Source: three-view drawing plus pictorial views. Frame: mm from the lowest corner of the part. Round coordinates to 2 decimals unless told otherwise and drop trailing zeros. Write each loop counter-clockwise with the first axis right and the second up, starting at its lowest first coordinate (ties: lowest second). Pieces come first, ordered by that corner, then holes. Notation, with made-up numbers: (54.25, 88.5) -> (112.25, 88.5) arc R12 cw to (112.25, 101.5) -> close; hole circle Ø7 at (1.25, 38). An arc over 180 degrees is marked (long way). Put each result on its own line as item: value.
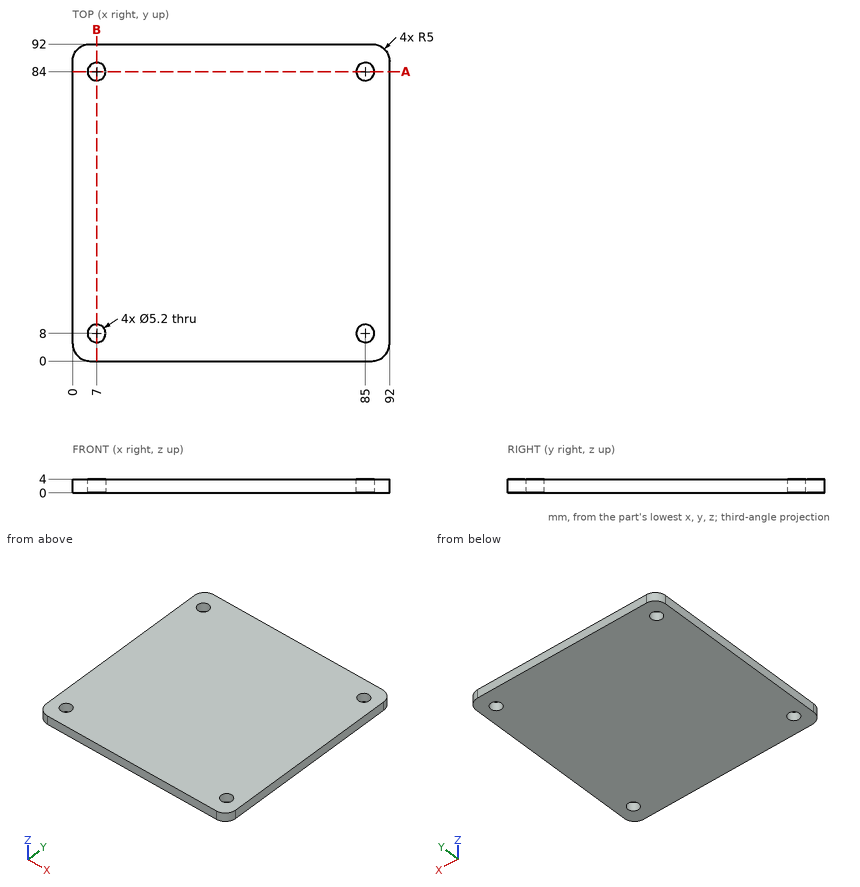
Q1. Cut plane A-A on y = 84. Output: boundary loops of the cut face in (x, z), and give its area (3 significant figures).
Ans:
outline: (0, 0) -> (4.4, 0) -> (4.4, 4) -> (0, 4) -> close; (9.6, 0) -> (82.4, 0) -> (82.4, 4) -> (9.6, 4) -> close; (87.6, 0) -> (92, 0) -> (92, 4) -> (87.6, 4) -> close
area: 326 mm^2
Q2. Pin query (flat end, axial travel): pin 1 (6 mm diameter, centred on x = 7, y = 84, fed in from -Z). Return the tip coordinate at first contact, or that it passes through.
Ans:
pin 1: stops at z = 0
Q3. Material intervals for line 1 (X direction, y = 84, z = 1.5); line 2 (Y direction, x = 7, z = 1.5); line 3 (X direction, y = 6, z = 2.75), sorted ascending. Write a range as [from, to].
Ans:
line 1: x = [0, 4.4], [9.6, 82.4], [87.6, 92]
line 2: y = [0, 5.4], [10.6, 81.4], [86.6, 92]
line 3: x = [0, 5.34], [8.66, 83.34], [86.66, 92]
Q4. Cut plane B-B on x = 7. Output: boundary loops of the cut face in (y, z).
Ans:
outline: (0, 0) -> (5.4, 0) -> (5.4, 4) -> (0, 4) -> close; (10.6, 0) -> (81.4, 0) -> (81.4, 4) -> (10.6, 4) -> close; (86.6, 0) -> (92, 0) -> (92, 4) -> (86.6, 4) -> close
